Input: part model. Units: mm. Frame: model coordinates. Coordinates: 2 decimals unless noted, no trailing zeros. Use a Markdown table: item, result. Add a question column.
from build123d import *

# Parameters (mm, degrees)
SKETCH1_W           = 208
SKETCH1_H           = 198
BOSS_EXTRUDE1_DEPTH = 1
INPUT_FOR_SPEAKER_R = 5
CUT_EXTRUDE1_DEPTH  = 10
SKETCH4_R           = 1.5
CUT_EXTRUDE2_DEPTH  = 1


with BuildPart() as part:
    # Sketch1 → Boss-Extrude1 (new body)
    with BuildSketch(Plane(origin=(0, 0, 0), x_dir=(1, 0, 0), z_dir=(0, 1, 0))):
        with Locations((104, 99)):
            Rectangle(SKETCH1_W, SKETCH1_H)
    extrude(amount=BOSS_EXTRUDE1_DEPTH)

    # Input for speaker → Cut-Extrude1 (cut)
    with BuildSketch(Plane(origin=(0, 1, 0), x_dir=(1, 0, 0), z_dir=(0, 1, 0))):
        with Locations(Location((104, 97.5, 0), (0, 0, 270))):
            Circle(INPUT_FOR_SPEAKER_R)
    extrude(amount=-CUT_EXTRUDE1_DEPTH, mode=Mode.SUBTRACT)

    # Sketch4 → Cut-Extrude2 (cut)
    with BuildSketch(Plane(origin=(0, 0, 0), x_dir=(-1, 0, 0), z_dir=(0, -1, 0))):
        with Locations(Location((-185, 98.797761971, 0), (0, 0, 90))):
            Circle(SKETCH4_R)
        with Locations(Location((-185, 71.557761971, 0), (0, 0, 90))):
            Circle(SKETCH4_R)
        with Locations(Location((-185, 53.4, 0), (0, 0, 90))):
            Circle(SKETCH4_R)
        with Locations(Location((-185, 26.16, 0), (0, 0, 90))):
            Circle(SKETCH4_R)
        with Locations(Location((-23, 26.16, 0), (0, 0, 270))):
            Circle(SKETCH4_R)
        with Locations(Location((-23, 53.4, 0), (0, 0, 270))):
            Circle(SKETCH4_R)
        with Locations(Location((-23, 71.557761971, 0), (0, 0, 270))):
            Circle(SKETCH4_R)
        with Locations(Location((-23, 98.797761971, 0), (0, 0, 270))):
            Circle(SKETCH4_R)
    extrude(amount=-CUT_EXTRUDE2_DEPTH, mode=Mode.SUBTRACT)


solid = part.part
1) Pull-direction query (Z, two-part tool) for faces 1 (the cylindrical face through (102.085, 0.507, -92.881)), 2 (the flat face through (103, 1, -122)); classes: pulls with the +Z half, pulls with the -Z half, needs draft (parallel to the pull), parting line crosses it, or undercut.
2) Contact query for a flat-ended pin moving along its axis: P1, Ø2.5, axis at x = 23, z = -98.8, coming from the -Y side. Output: stop coordinate, or through.
3) Material intervals for L1, parallel to Z at x = 185, y = 0.65; L2, parallel to X at y = 0.85, z = -26.16; L3, parallel to X at y = 0.4, z = -97.5, sorted ascending.
Computed:
| question | item | result |
|---|---|---|
| 1 | face 1 | undercut |
| 1 | face 2 | needs draft |
| 2 | P1 | passes through |
| 3 | L1 | z = -198 to -100.3, -97.3 to -73.06, -70.06 to -54.9, -51.9 to -27.66, -24.66 to 0 |
| 3 | L2 | x = 0 to 21.5, 24.5 to 183.5, 186.5 to 208 |
| 3 | L3 | x = 0 to 22.25, 23.75 to 99, 109 to 184.25, 185.75 to 208 |
